Source: three-view drawing plus pictorial views. Frame: mm from the lowest corner of the part. Give positions to 0.01 mm unless a question says otherwise; leave off trailing zeros. Order: outer loops, then holes, each group sorted by start corner. A loop starts at its lowest first (then second) coordinate and runs counter-clockwise, first axis right, second up. Notation, with made-up numbers: (17.5, 12) -> (25.5, 12) arc R17 cw to (25.5, 39) -> close; hole circle Ø2 at (76.25, -7.75). An arc over 180 degrees is marked (long way). Write item = value, one per line.
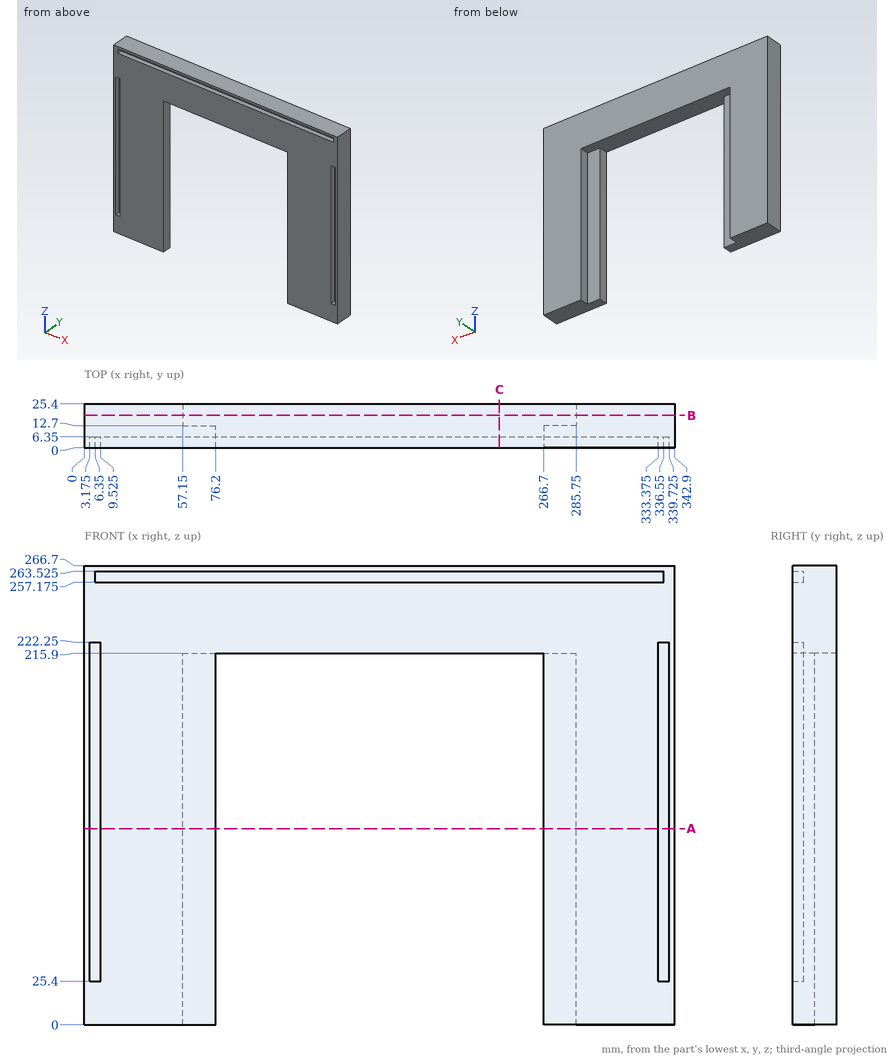
1) Section query B-B (y = 18.75). Output: boundary loops of the cut face in (x, z).
Check sheet entries:
outline = (0, 0) -> (57.15, 0) -> (57.15, 215.9) -> (285.75, 215.9) -> (285.75, 0) -> (342.9, 0) -> (342.9, 266.7) -> (0, 266.7) -> close
2) Section query C-C (x = 241). Output: boundary loops of the cut face in (y, z) (3 decimals).
Check sheet entries:
outline = (0, 215.9) -> (25.4, 215.9) -> (25.4, 266.7) -> (0, 266.7) -> (0, 263.525) -> (6.35, 263.525) -> (6.35, 257.175) -> (0, 257.175) -> close
3) Line query: line 1 (X direction, y = 2.25, z = 93) (3 decimals); line 2 (Z direction, x = 261.5, y = 4.75) (3 decimals); line 3 (Z direction, x = 302, y = 4.5) (3 decimals). Output: solid intervals per line, ascending. Write a range as from..to.
Check sheet entries:
line_1 = 0..3.175, 9.525..76.2, 266.7..333.375, 339.725..342.9
line_2 = 215.9..257.175, 263.525..266.7
line_3 = 0..257.175, 263.525..266.7
4) First-contact query: P1, Ø3, axis at x = 7.5, z = 79.5, coming from the -Y side; P2, Ø8, axis at x = 67, z = 52, coming from the +Y side. Flat tips, straight axial feed; report the tip coordinate or a pass-through.
Check sheet entries:
P1 = 6.35
P2 = 12.7
5) Section query A-A (z = 114). Output: boundary loops of the cut face in (x, y) (3 decimals), plus the area to 3 significant figures.
Check sheet entries:
outline = (0, 0) -> (3.175, 0) -> (3.175, 6.35) -> (9.525, 6.35) -> (9.525, 0) -> (76.2, 0) -> (76.2, 12.7) -> (57.15, 12.7) -> (57.15, 25.4) -> (0, 25.4) -> close; (266.7, 0) -> (333.375, 0) -> (333.375, 6.35) -> (339.725, 6.35) -> (339.725, 0) -> (342.9, 0) -> (342.9, 25.4) -> (285.75, 25.4) -> (285.75, 12.7) -> (266.7, 12.7) -> close
area = 3,310 mm²
